```python
from build123d import *

# Parameters (mm, degrees)
F1_DEPTH = 63.5
F2_DEPTH = 25.4
F3_DEPTH = 7.9375
F0_W     = 25.4
F0_H     = 28.575
F5_R     = 6.35


with BuildPart() as f1:
    # F0 (on Front) → F1 (new body, symmetric)
    with BuildSketch(Plane.XZ):
        Polygon((22.225, 9.525), (-41.275, 9.525), (-41.275, -9.525), (41.275, -9.525), (41.275, 9.525), align=None)
    extrude(amount=F1_DEPTH, both=True)

    # F0 (on Front) → F2 (join, symmetric)
    with BuildSketch(Plane.XZ):
        with BuildLine():
            Line((22.225, 27.1272), (22.225, 9.525))
            Line((22.225, 9.525), (41.275, 9.525))
            Line((41.275, 9.525), (41.275, 27.1272))
            ThreePointArc((41.275, 27.1272), (45.92468, 38.35252), (57.15, 43.0022))
            Line((57.15, 43.0022), (60.325, 43.0022))
            Line((60.325, 43.0022), (60.325, 62.0522))
            Line((60.325, 62.0522), (57.15, 62.0522))
            add(Edge.make_bspline(
                [(28.136121, 46.568148), (37.807414, 51.729499), (47.478707, 56.890849), (57.15, 62.0522)],
                knots=[78.677179, 78.677179, 78.677179, 78.677179, 111.564275, 111.564275, 111.564275, 111.564275], degree=3))
            ThreePointArc((28.136121, 46.568148), (23.735442, 37.28707), (22.225, 27.1272))
        make_face()
        Polygon((60.325, 66.675), (60.325, 62.0522), (60.325, 43.0022), (60.325, 38.1), (85.725, 38.1), (85.725, 66.675), align=None)
    extrude(amount=F2_DEPTH, both=True)

    # F0 (on Front) → F3 (join, symmetric)
    with BuildSketch(Plane.XZ):
        with BuildLine():
            add(Edge.make_bspline(
                [(-41.275, 9.525), (-18.13796, 21.872716), (4.999081, 34.220432), (28.136121, 46.568148)],
                knots=[0, 0, 0, 0, 78.677179, 78.677179, 78.677179, 78.677179], degree=3))
            Line((-41.275, 9.525), (22.225, 9.525))
            Line((22.225, 9.525), (22.225, 27.1272))
            ThreePointArc((22.225, 27.1272), (23.735442, 37.28707), (28.136121, 46.568148))
        make_face()
    extrude(amount=F3_DEPTH, both=True)

    # F0 (on Front) → F4 (revolve)
    with BuildSketch(Plane.XZ):
        with Locations((98.425, 52.3875)):
            Rectangle(F0_W, F0_H)
    revolve(axis=Axis((85.725, 0, 52.3875), (0, 0, 1)))

    # F5
    f5_edges = [f1.edges().sort_by_distance(p)[0] for p in [
        (41.275, -63.5, 0),
        (-41.275, -63.5, 0),
        (-41.275, 63.5, 0),
        (41.275, 63.5, 0),
    ]]
    fillet(f5_edges, radius=F5_R)


solid = f1.part
```
Work out the finished part from the listing and answer in its coordinate system (mm). A direction names the side the tool comes from. Give positions to 0.01 mm unless a question says otherwise; leave off trailing zeros. Loops run counter-clockwise (first coordinate to the right, second up) from the corner with the lowest first, then second, coordinate; pieces in that order, holes last. Notation, with made-up numbers: (-25, 12.25) -> (-2, 12.25) arc R16 cw to (-2, 17.25) -> close; hole circle Ø2 at (36, 3). An arc over 180 degrees is marked (long way). One line per question, with ' | ' between items. Start each with the question number.
1) Each of these flat-tipped pins is pushed along its axis until it touches: pin 1 (4 mm diameter, centred on y = 11, z = 41.5, fed in from -X); pin 2 (18.5 mm diameter, centred on x = -6.5, z = 29.5, fed in from +Y); pin 3 (5 mm diameter, centred on x = 43, z = 27.5, fed in from +Y); pin 4 (2 mm diameter, centred on x = 88.5, z = 36.5, fed in from -Y). Where does it stop, or does it pass through?
2) Straight lines are drawn through the part: L1, parallel to Y at x = -7, z = 25.5; L2, parallel to Z at x = -26.5, y = -26.5 (3 decimals); L3, parallel to Z at x = 97.5, y = 18.5 (3 decimals). For each, find the intervals that lie inside material, in ascending order.
3) Section C-C, the plane x = 93 is taken. Determine the outline of the cut face in (y, z) (3 decimals).
4) Section A-A, the plane z = -3 is taken. Determine the outline of the cut face in (x, y) (3 decimals), then the cut area to 3 significant figures.
5) Section B-B, the plane y = -40 is taken. Determine the outline of the cut face in (x, z) (3 decimals), then the cut area to 3 significant figures.
6) Determine the mould class of faces 1 (the face through (60.325, 0, 41)), 2 (the face through (22.225, 17, 18)), 3 (the face through (54, -25.4, 45)) for opening direction X: +X half, -X half, draft (parallel to the pull), parting line (faces both ways), or undercut.
7) For faces 4 (the face through (60.325, 0, 64)), 5 (the face through (1, -7.938, 23)), 6 (the face through (86, 0, 38.1)), 7 (the face through (23.78, 16.55, 37.43)), determine the directions among +Z, -Z, +X, -X, +Y, -Y from which every point of the face is accessible in a straight line to the end or side of a thin tool.
Resolved:
1) pin 1: x = 24.49 | pin 2: y = 7.94 | pin 3: y = 25.4 | pin 4: through
2) L1: -7.94 to 7.94 | L2: -9.525 to 9.525 | L3: 38.1 to 66.675
3) outline: (-24.336, 38.1) -> (24.336, 38.1) -> (24.336, 66.675) -> (-24.336, 66.675) -> close
4) outline: (-41.275, -57.15) arc R6.35 ccw to (-34.925, -63.5) -> (34.925, -63.5) arc R6.35 ccw to (41.275, -57.15) -> (41.275, 57.15) arc R6.35 ccw to (34.925, 63.5) -> (-34.925, 63.5) arc R6.35 ccw to (-41.275, 57.15) -> close | area: 10,400 mm2
5) outline: (-41.275, -9.525) -> (41.275, -9.525) -> (41.275, 9.525) -> (-41.275, 9.525) -> close | area: 1,570 mm2
6) face 1: undercut | face 2: -X half | face 3: draft
7) face 4: +Z, -X, +Y, -Y | face 5: +Z, -X, -Y | face 6: -Z, +X, +Y, -Y | face 7: +Z, -X, +Y
